CAD build for the part. Positions are in the model's coordinates, mm. A direction names the side the tool comes from. Round coordinates to 2 decimals unless told otherwise and drop trailing zeros. Loops run counter-clockwise (first coordinate to the right, second up) from the corner with the lowest first, then second, coordinate; pieces in that order, holes last.
Autodesk Inventor part; units mm, degrees
ref_plane "YZ Plane" through (0, 0, 0) normal (1, 0, 0) x (0, 1, 0)
ref_plane "XZ Plane" through (0, 0, 0) normal (0, 1, 0) x (-1, 0, 0)
ref_plane "XY Plane" through (0, 0, 0) normal (0, 0, 1) x (1, 0, 0)
sketch "Sketch1" plane through (0, 0, 0) normal (0, 1, 0) x (-1, 0, 0)
  line L0 (42.8447, -6.952) -> (51.5823, -6.952)
  line L1 (51.5823, -6.952) -> (51.5823, -0.4834)
  line L2 (51.5823, -0.4834) -> (42.8447, -0.4834)
  line L3 (42.8447, -0.4834) -> (42.8447, -6.952)
  line L4 (-0.7823, -48.4843) -> (7.9553, -48.4843)
  line L5 (7.9553, -48.4843) -> (7.9553, -42.0157)
  line L6 (7.9553, -42.0157) -> (-0.7823, -42.0157)
  line L7 (-0.7823, -42.0157) -> (-0.7823, -48.4843)
  line L8 (7.9451, -6.952) -> (-0.7823, -6.952)
  line L9 (-0.7823, -6.952) -> (-0.7823, 1.7754)
  line L10 (-0.7823, 1.7754) -> (7.9451, 1.7754)
  line L11 (7.9451, 1.7754) -> (7.9451, -6.952)
  line L12 (42.8549, -50.7432) -> (42.8549, -42.0157)
  line L13 (51.5823, -50.7432) -> (42.8549, -50.7432)
  line L14 (51.5823, -42.0157) -> (51.5823, -50.7432)
  line L15 (42.8549, -42.0157) -> (51.5823, -42.0157)
  line L16 (42.8447, -2.5883) -> (7.935, -2.5883)
  line L17 (42.8549, -42.0157) -> (42.8549, -46.3795)
  line L18 (42.8549, -46.3795) -> (7.9451, -46.3795)
  line L19 (42.8549, -42.0157) -> (47.2186, -42.0157)
  line L20 (7.9451, -6.952) -> (3.5865, -6.952)
  line L21 (3.5865, -6.952) -> (3.5865, -42.0157)
  line L22 (12.309, -38.1974) -> (38.491, -38.1974)
  line L23 (38.491, -38.1974) -> (38.491, -10.7703)
  line L24 (38.491, -10.7703) -> (12.309, -10.7703)
  line L25 (12.309, -10.7703) -> (12.309, -38.1974)
  line L26 (47.2135, -10.7703) -> (60.3097, -10.7703)
  line L27 (60.3097, -10.7703) -> (60.3097, -38.1974)
  line L28 (60.3097, -38.1974) -> (47.2186, -38.1974)
  line L29 (47.2135, -6.952) -> (47.2135, -10.7703)
  line L30 (47.2186, -38.1974) -> (47.2186, -42.0157)
  line L31 (47.2135, -6.952) -> (51.5823, -6.952)
  line L32 (49.4004, -13.4933) -> (58.1279, -13.4933)
  line L33 (58.1279, -13.4933) -> (58.1279, -35.1517)
  line L34 (58.1279, -35.1517) -> (49.4004, -35.1517)
  line L35 (49.4004, -35.1517) -> (49.4004, -13.4933)
  circle A0 centre (47.2186, -2.5883) radius 0.6982
  circle A1 centre (3.5814, -2.5883) radius 0.6982
  circle A2 centre (3.5814, -46.3795) radius 0.6982
  circle A3 centre (47.2186, -46.3795) radius 0.6982
  point P0 (0, 0)
  point P1 (25.4, -24.4839)
  point P2 (3.5865, -6.952)
  point P3 (7.9553, -46.3795)
  point P4 (7.9451, -2.5883)
  point P5 (47.2186, -42.0157)
  dimension "d2" = 8.7376
  dimension "d6" = 360
  dimension "d10" = 360
  dimension "d19" = 5.7909
  dimension "d20" = 5.7909
  dimension "d21" = 13.0912
  dimension "d29" = 1.3964
  dimension "d32" = 360
  dimension "d38" = 43.6372
extrude "Extrusion3" add sketch "Sketch1" along normal blind 2.54
fillet "Fillet4" radius 3.175 14 edges at (-51.5823, 1.27, -0.4834) (-42.8447, 1.27, -0.4834) (-51.5823, 1.27, -6.952) (-7.9451, 1.27, 1.7754) (0.7823, 1.27, 1.7754) (0.7823, 1.27, -6.952) (0.7823, 1.27, -42.0157) (0.7823, 1.27, -48.4843) (-7.9553, 1.27, -48.4843) (-42.8549, 1.27, -50.7432) (-51.5823, 1.27, -50.7432) (-51.5823, 1.27, -42.0157) (-60.3097, 1.27, -38.1974) (-60.3097, 1.27, -10.7703)
equation "\"BendRadius\" = Thickness"
equation "\"BendReliefWidth\" = Thickness"
equation "\"BendReliefDepth\" = 0.5 * Thickness"
equation "\"CornerReliefSize\" = 4 * Thickness"
equation "\"MinimumRemnant\" = 2 * Thickness"
equation "\"TransitionRadius\" = BendRadius"
equation "\"JacobiRadiusSize\" = BendRadius"
equation "\"GapSize\" = Thickness"
properties part number "PixfalconHolder"
Item 1: Cut at B-B, the plane z = -18.5. Give the cut face in (x, y), plus the area to 3 significant figures.
Answers follow:
outline: (-60.31, 0) - (-58.13, 0) - (-58.13, 2.54) - (-60.31, 2.54) - close; (-49.4, 0) - (-38.49, 0) - (-38.49, 2.54) - (-49.4, 2.54) - close; (-12.31, 0) - (-3.59, 0) - (-3.59, 2.54) - (-12.31, 2.54) - close
area: 55.4 mm2
Item 2: Cut at C-C, the plane z = -37. Give the cut face in (x, y), plus the area to 3 significant figures.
Answers follow:
outline: (-59.62, 0) - (-38.49, 0) - (-38.49, 2.54) - (-59.62, 2.54) - close; (-12.31, 0) - (-3.59, 0) - (-3.59, 2.54) - (-12.31, 2.54) - close
area: 75.8 mm2
Item 3: Probe line 1 (X direction, y = 1.7, z = -27); line 2 (Z direction, x = -24.5, y = 1.75); line 3 (Z direction, x = -2.5, y = 1.15). List the from-to ranges inside material, lowest first.
Answers follow:
line 1: x = -60.31 to -58.13, -49.4 to -38.49, -12.31 to -3.59
line 2: z = -46.38 to -38.2, -10.77 to -2.59
line 3: z = -48.48 to -42.02, -6.95 to 1.78
Item 4: Cut at D-D, the plane y = 0.9. State how many separate pieces and enclosed holes the cut face has, plus the area to 3 significant figures.
Answers follow:
separate pieces: 1
enclosed holes: 6
area: 1,520 mm2
Item 5: Two-plate mould, pull along Z, no slides. Class faces 1 (the flat face through (-43, 2.54, -24)), 2 (the cylindrical face through (-59.404, 1.252, -37.243)), 3 (the cylindrical face through (-46.665, 1.252, -45.955)): released by +Z, released by -Z, zero draft, split by the parting line, or undercut.
Answers follow:
face 1: zero draft
face 2: released by -Z
face 3: undercut
Item 6: Cut at A-A, the plane x = -19. Give the cut face in (y, z), plus the area to 3 significant figures.
Answers follow:
outline: (0, -46.38) - (2.54, -46.38) - (2.54, -38.2) - (0, -38.2) - close; (0, -10.77) - (2.54, -10.77) - (2.54, -2.59) - (0, -2.59) - close
area: 41.6 mm2
Item 7: Flat gauge pins, fed straight in: P1, Ø0.8, axis at y = 1.5, z = -26, coming from the +X side; P2, Ø1.3, axis at x = -30, y = 1, coming from the +Z side; P3, Ø0.6, axis at y = 1, z = -47, coming from the +X side. Where does each tip first touch, or does it go through?
Answers follow:
P1: stops at x = -3.59
P2: stops at z = -2.59
P3: stops at x = 0.46
Item 8: 3-axis set-ups, long thin cutter, end or side, ignore diameter. For faces 4 (the cylindrical face through (-43.98, 1.25, -1.08)), 5 (the flat face through (-3.586, 1, -24)), 6 (the cylindrical face through (-50.628, 1.252, -42.921)), 7 (the flat face through (-26, 1, -46.38)), 8 (the flat face through (-47, 1, -0.483)): which of +Z, -Z, +X, -X, +Y, -Y reach the whole face in a straight line?
Answers follow:
face 4: +Z, +Y, -Y
face 5: +X, +Y, -Y
face 6: -X, +Y, -Y
face 7: -Z, +Y, -Y
face 8: +Z, -X, +Y, -Y
